Design review of the part shown in the three views and the two pictorial views. Dimensions are in mm from the part's minimum x, y and z. Round coordinates to 2 decimals unless told otherwise and drop trailing zeros. Write each loop counter-clockwise with the first axis right and the second up, starting at its lowest first coordinate (ties: lowest second). Pieces come first, ordered by that corner, then holes. Notation, with made-up numbers: (-15, -7.5) -> (33, -7.5) arc R15 ccw to (33, -3.5) -> close; hole circle Ø6 at (88, -15.5). An arc over 180 degrees is marked (long way). Answer as a JSON object with one key per item and string values. Group by question number.
1) We need section B-B, the plane x = 20. Count the separate pieces of the cut face and the enclosed holes in it, then the cut area to 3 significant figures.
2) To check wall thickness, follow probe 1 along Z at (x, y) = (23, 32) (3 decimals); probe 2 along X at (y, z) = (34, 32.5); probe 3 along X at (y, z) = (8.5, 35). State the ranges of each line that lie inside material, in increasing order. Write a range as [from, to].
3) We need section D-D, the plane z = 3.5. Write out the cut boundary in (x, y) (3 decimals).
4) Insertion check: pin 1 Ø1 at (x, z) = (9.5, 9) entering from -Y; pin 2 Ø4.5 at (x, z) = (22.225, 30.48) entering from -Y; pin 3 Ø4 at (y, z) = (5.5, 36.5) entering from -X; pin 4 Ø5 at (x, z) = (35.5, 18) entering from +Y. Each pin has a flat end and moves straight along its axis. Give the tip position at first contact, or say it passes through.
5) We need section A-A, the plane z = 30.48. Write out the cut boundary in (x, y) (3 decimals).
6) Mouldability with a two-part tool opening along Y and no side actions: class the marked faces 1, 2 and 3 as pulls with the +Y half, pulls with the -Y half, needs draft (parallel to the pull), parting line crosses it, or undercut.
7) We need section C-C, the plane z = 26. Write out the cut boundary in (x, y) (3 decimals), then the cut area to 3 significant figures.
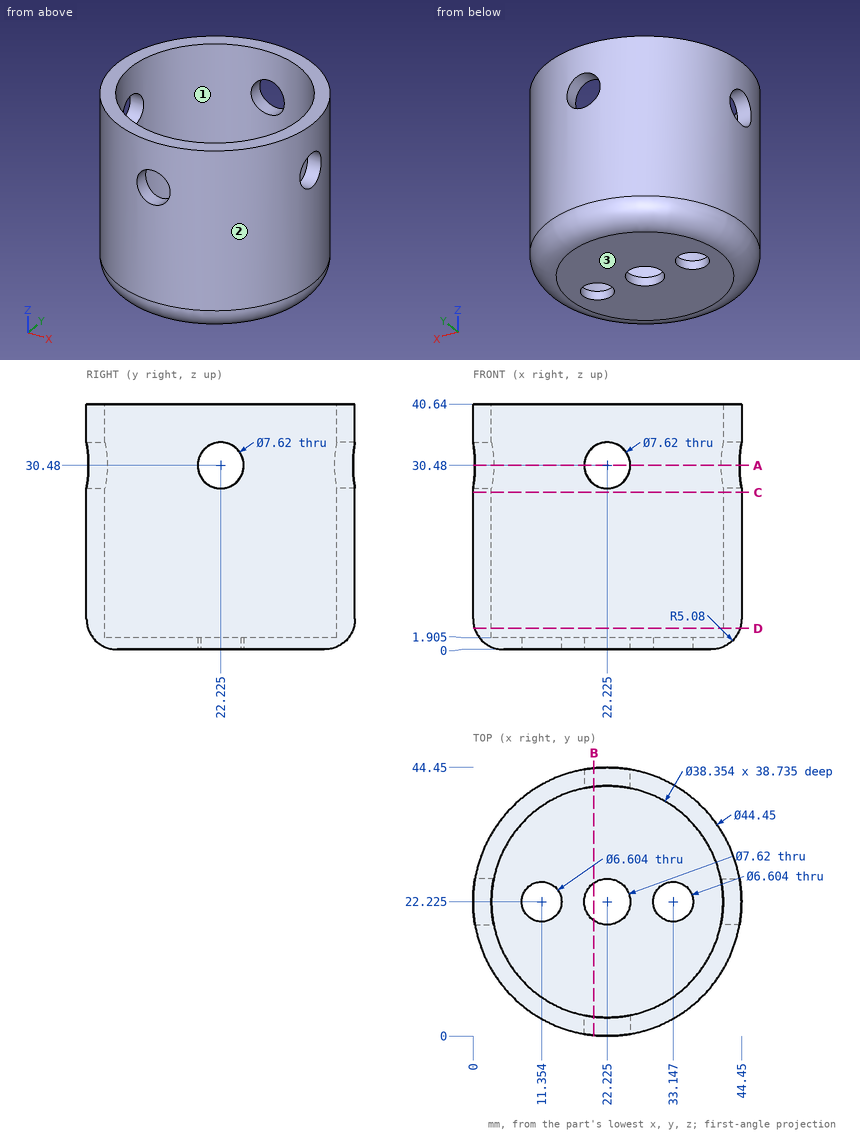
Here are the results:
{
 "1": {"separate pieces": "4", "enclosed holes": "0", "area": "261 mm^2"},
 "2": {"probe 1": "z = [0, 1.905]", "probe 2": "x = [3.38, 7.09], [37.36, 41.07]", "probe 3": "x = [4.74, 8.83], [35.62, 39.71]"},
 "3": {"outline": "circle Ø43.946 at (22.225, 22.225); hole circle Ø38.354 at (22.225, 22.225)"},
 "4": {"pin 1": "stops at y = 3.66", "pin 2": "passes through", "pin 3": "stops at x = 5.58", "pin 4": "stops at y = 41.66"},
 "5": {"outline": "(0.329, 18.415) arc R22.225 ccw to (18.415, 0.329) -> (18.415, 3.43) arc R19.177 cw to (3.43, 18.415) -> close; (0.329, 26.035) -> (3.43, 26.035) arc R19.177 cw to (18.415, 41.02) -> (18.415, 44.121) arc R22.225 ccw to start; (26.035, 0.329) arc R22.225 ccw to (44.121, 18.415) -> (41.02, 18.415) arc R19.177 cw to (26.035, 3.43) -> close; (26.035, 41.02) arc R19.177 cw to (41.02, 26.035) -> (44.121, 26.035) arc R22.225 ccw to (26.035, 44.121) -> close"},
 "6": {"face 1": "undercut", "face 2": "parting line crosses it", "face 3": "needs draft"},
 "7": {"outline": "circle Ø44.45 at (22.225, 22.225); hole circle Ø38.354 at (22.225, 22.225)", "area": "396 mm^2"}
}
